```python
from build123d import *

# Parameters (mm, degrees)
CUT_EXTRUDE_2_DEPTH      = 57.160484328
CUT_EXTRUDE_2_DEPTH_BACK = 57.160484328
SKETCH_2_OUTSIDE_W       = 49.234
SKETCH_2_OUTSIDE_H       = 94.234
SKETCH_2_OUTSIDE_W_2     = 20
SKETCH_2_OUTSIDE_H_2     = 75
EXTRUDE_1_DEPTH          = 11
EXTRUDE_1_DEPTH_BACK     = 11
SKETCH_4_W               = 22
SKETCH_4_H               = 8
SKETCH_5_R               = 1.7
CUT_EXTRUDE_3_DEPTH      = 59.051701095


with BuildPart() as part:
    # Sketch 1 → Revolve 1 (revolve)
    with BuildSketch(Plane.XY, mode=Mode.PRIVATE) as revolve_1_sk:
        Polygon((2.5, 0), (15, 0), (15, 42), (5, 42), (5, 52), (3, 52), (3, 42), (0, 42), (0, 0), (0, -23), (0.2, -23), (2.5, -19.016283143), align=None)
    revolve(revolve_1_sk.sketch.rotate(Axis((0, 0, 0), (0, 1, 0)), 90), axis=Axis((0, 0, 0), (0, 1, 0)))

    # Sketch 2 outside → Cut-Extrude 2 (cut, two sides: drawn at the far end of the back side and taken through both)
    with BuildSketch(Plane.XY.offset(-CUT_EXTRUDE_2_DEPTH_BACK)):
        with Locations((0, 14.5)):
            Rectangle(SKETCH_2_OUTSIDE_W, SKETCH_2_OUTSIDE_H)
        with Locations((0, 14.5)):
            Rectangle(SKETCH_2_OUTSIDE_W_2, SKETCH_2_OUTSIDE_H_2, mode=Mode.SUBTRACT)
    extrude(amount=CUT_EXTRUDE_2_DEPTH + CUT_EXTRUDE_2_DEPTH_BACK, mode=Mode.SUBTRACT)

    # Sketch 4 → Extrude 1 (add, two sides: drawn at the far end of the back side and taken through both)
    with BuildSketch(Plane.XY.offset(-EXTRUDE_1_DEPTH_BACK)):
        with Locations((0, -13)):
            Rectangle(SKETCH_4_W, SKETCH_4_H)
    extrude(amount=EXTRUDE_1_DEPTH + EXTRUDE_1_DEPTH_BACK)

    # Sketch 5 → Cut-Extrude 3 (cut, through all)
    with BuildSketch(Plane(origin=(10, 0, 0), x_dir=(0, 0, -1), z_dir=(1, 0, 0))):
        with Locations((-6, 32)):
            Circle(SKETCH_5_R)
        with Locations((6, 32)):
            Circle(SKETCH_5_R)
    extrude(amount=-CUT_EXTRUDE_3_DEPTH, mode=Mode.SUBTRACT)


solid = part.part
```
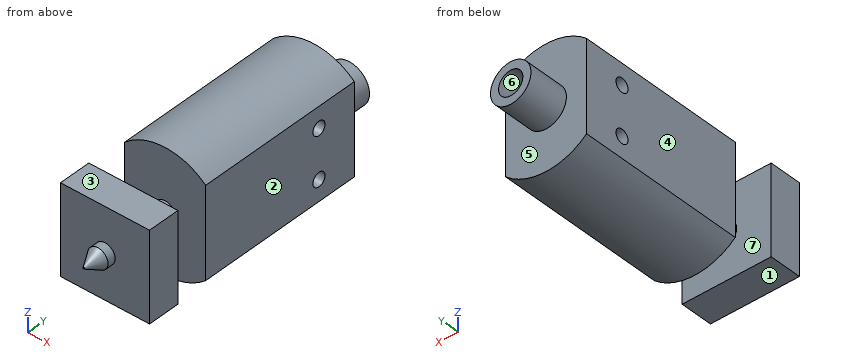
The model under review builds one solid part; all positions refer to its coordinate system, in mm. Face numbers are marked on the shaded views. A direction names the side the tool comes from. Give positions to 0.01 mm unless a question says otherwise; leave off trailing zeros. Write each loop counter-clockwise with the first axis right and the second up, starting at its lowest first coordinate (ties: lowest second). Pieces come first, ordered by that corner, then holes. Notation, with made-up numbers: M 20.5,-19 L 74.5,-19 A29 cw 74.5,6 Z; hole C -16,5.5 d6. An arc over 180 degrees is marked long. Write each question's results on one line, items separated by ' | '. Start each with the question number.
1. Mouldability with a two-part tool opening along Y and no side actions: class the marked faces 5, 6 and 7 as released by +Y, released by -Y, zero draft, split by the parting line, or undercut.
2. We need section B-B (x = 8). Write out the cut boundary in (y, z), and give its area (3 significant figures).
3. For probe 1 along Y at (x, z) = (5.75, 6); probe 2 along Y at (x, z) = (-3.75, 9); probe 3 along X at (y, z) = (45, 0), list the stretches that pass through material, from the lowest coordinate up. Write a range as [from, to].
4. We need section A-A (y = 32). Write out the cut boundary in (x, z).
5. For the marked faces 1, 2, 3 and 4, list the 3-axis set-ups (+Z, -Z, +X, -X, +Y, -Y) from which the entire face can be reached by the end or side of a thin tool; tool diameter is ignored.
6. We need section C-C (z = 9). Write out the cut boundary in (x, y), and give its area (3 significant figures).
7. We need section D-D (z = -6). Write out the cut boundary in (x, y).
8. Insertion check: pin 1 Ø2.5 at (x, y) = (4, -13.5) entering from +Z; pin 2 Ø4.5 at (y, z) = (32, 6) entering from -X; pin 3 Ø1 at (y, z) = (-5.5, 1) entering from -X. Each pin has a flat end and moves straight along its axis. Give the tip position at first contact, or say it passes through.
Results found:
1) face 5: released by +Y | face 6: zero draft | face 7: undercut
2) outline: M -17,-11 L -9,-11 L -9,11 L -17,11 Z; M 0,-12.69 L 42,-12.69 L 42,12.69 L 0,12.69 Z; hole C 32,-6 d3.4; hole C 32,6 d3.4 | area: 1,220 mm^2
3) probe 1: y = [-17, -9], [0, 30.3], [33.7, 42] | probe 2: y = [-17, -9], [0, 42] | probe 3: x = [-5, -3], [3, 5]
4) outline: M -10,-11.18 A15 ccw 10,-11.18 L 10,-7.7 L -10,-7.7 Z; M -10,-4.3 L 10,-4.3 L 10,4.3 L -10,4.3 Z; M -10,7.7 L 10,7.7 L 10,11.18 A15 ccw -10,11.18 Z
5) face 1: -Z, +X, -X, -Y | face 2: +Z, -Z, +X, +Y | face 3: +Z, +X, -X, -Y | face 4: +Z, -Z, -X, +Y
6) outline: M -11,-17 L 11,-17 L 11,-9 L -11,-9 Z; M -10,0 L 10,0 L 10,42 L -10,42 Z | area: 1,020 mm^2
7) outline: M -11,-17 L 11,-17 L 11,-9 L -11,-9 Z; M -10,0 L 10,0 L 10,30.3 L -10,30.3 Z; M -10,33.7 L 10,33.7 L 10,42 L -10,42 Z
8) pin 1: stops at z = 11 | pin 2: stops at x = -10 | pin 3: stops at x = -2.45
